Verification items for the finished model (mm, model axes). A direction names the side the tool comes from. Give positions to 0.01 mm unless a question says otherwise; leave off trailing zeros. Order: outer loops, then holes, each group sorted by start corner. A loop starts at its lowest first (then second) coordinate and runs counter-clockwise, first axis right, second up.
from build123d import *

# Parameters (mm, degrees)
F4_DEPTH      = 6
F4_DEPTH_BACK = 6


with BuildPart() as f1:
    # F0 (on Front) → F1 (revolve)
    with BuildSketch(Plane.XZ):
        Polygon((0, 8), (-6.5, 8), (-6.5, 0), (-4, 0), (-4, -99.235), (-3.235, -100), (0, -100), align=None)
    revolve(axis=Axis((0, 0, -46), (0, 0, -1)))

    # F3 (on offset) → F4 (cut, two sides)
    with BuildSketch(Plane.XY.offset(8)) as f4_sk:
        Polygon((3, -1.732051), (3, 1.732051), (0, 3.464102), (-3, 1.732051), (-3, -1.732051), (0, -3.464102), align=None)
    extrude(amount=-F4_DEPTH, mode=Mode.SUBTRACT)
    extrude(f4_sk.sketch, amount=-F4_DEPTH_BACK, mode=Mode.SUBTRACT)


solid = f1.part
(1) Section check B-B, the plane z = -13.5. Enter the section's corners in (x, y), then the cut area to 3 significant figures.
Solved:
outline: circle Ø8 at (0, 0)
area: 50.3 mm2
(2) Set-up check for faces 1 (the flat face through (1.5, 2.6, 5)), 2 (the cylindrical face through (5.158, -3.955, 3.944)): record each of +Z, -Z, +X, -X, +Y, -Y from which the full face is reachable in a straight line by a thin tool's end or side.
Solved:
face 1: +Z
face 2: +Z, -Z
(3) Scan lines: line 1 (Z direction, x = 0.75, y = 2.75); line 2 (X direction, y = -0.25, z = -60); line 3 (Z direction, x = -5.5, y = -1.75). Record each from-to range of solid material in increasing order.
Solved:
line 1: z = -100 to 2
line 2: x = -3.99 to 3.99
line 3: z = 0 to 8
(4) Go/stop test with flat-tipped pins: pin 1 (6 mm diameter, centred on y = -1, z = -50, fed in from -X); pin 2 (4 mm diameter, centred on x = 2, z = -37, fed in from -Y); pin 3 (1 mm diameter, centred on y = -0.5, z = 6, fed in from +X); pin 4 (1.8 mm diameter, centred on x = 0, y = -0.5, fed in from +Z). Record where each tip stops, or that it passes through.
Solved:
pin 1: stops at x = -4
pin 2: stops at y = -4
pin 3: stops at x = 6.5
pin 4: stops at z = 2
(5) Release check for a two-part mould opening along Y. For faces 3 (the flat face through (0, 0, 2)), 4 (the cylindrical face through (0.867, -3.905, -50.312)), 5 (the flat face through (-3, 0, 5)), 6 (the flat face through (-3, 3, 0)) record: pulls with the +Y half, pulls with the -Y half, needs draft (parallel to the pull), parting line crosses it, or undercut.
Solved:
face 3: undercut
face 4: parting line crosses it
face 5: undercut
face 6: needs draft
(6) Section check A-A, the plane y = 0. Enter the section's corners in (x, z) (3 decimals), then the cut area to 3 significant figures.
Solved:
outline: (-6.5, 0) - (-4, 0) - (-4, -99.235) - (-3.235, -100) - (3.235, -100) - (4, -99.235) - (4, 0) - (6.5, 0) - (6.5, 8) - (3, 8) - (3, 2) - (-3, 2) - (-3, 8) - (-6.5, 8) - close
area: 867 mm2
(7) Section check C-C, the plane x = 5.25. Enter the section's corners in (y, z), then the cut area to 3 significant figures.
Solved:
outline: (-3.83, 0) - (3.83, 0) - (3.83, 8) - (-3.83, 8) - close
area: 61.3 mm2
